Source: CAD feature listing. Evaluate the final solid. Frame: model axes, mm. A direction names the side the tool comes from. Coordinates: 2 decimals unless noted, no trailing zeros. Write each loop counter-clockwise with the first axis right and the second up, starting at its lowest first coordinate (ties: lowest second). Pieces come first, ordered by that corner, then holes. Notation, with made-up numbers: (-23, -0.5) - (22, -0.5) arc R38 cw to (22, 37.5) - close; hole circle Ø7 at (15, 81.5). An arc over 180 degrees is marked (long way). One line per question, with ' | ' between items.
from build123d import *

# Parameters (mm, degrees)
SCHIZZO1_R                   = 10
SCHIZZO1_R_2                 = 1.2
ESTRUSIONE_ESTRUSIONE1_DEPTH = 6
SCHIZZO2_R                   = 5
ESTRUSIONE_ESTRUSIONE2_DEPTH = 53
SCHIZZO9_W                   = 4
SCHIZZO9_H                   = 2.3
SMUSSO3_SIZE                 = 0.3
FORO_8_1_8_1_1_D             = 8.1
FORO_8_1_8_1_1_DEPTH         = 2
FORO_8_1_8_1_1_TIP           = 2.433485507
SMUSSO5_SIZE                 = 0.5
TAGLIO_ESTRUSIONE1_START     = -29
TAGLIO_ESTRUSIONE1_DEPTH     = 29
PREFORO_DA_MASCHIARE_M3_1_D  = 2.5
SMUSSO4_SIZE                 = 0.3
FORO_8_1_8_1_2_D             = 8.1
FORO_8_1_8_1_2_DEPTH         = 2.5
FORO_8_1_8_1_2_TIP           = 2.433485507
SCHIZZO17_W                  = 1.3
SCHIZZO17_H                  = 4.4
RACCORDO1_R                  = 0.2
SCHIZZO18_W                  = 0.2
SCHIZZO18_H                  = 1.1


with BuildPart() as part:
    # Schizzo1 → Estrusione-Estrusione1 (new body)
    with BuildSketch(Plane(origin=(0, 0, 0), x_dir=(1, 0, 0), z_dir=(0, 1, 0))):
        with Locations(Location((0, 0, 0), (0, 0, 270))):
            Circle(SCHIZZO1_R)
        with Locations(Location((0, 8, 0), (0, 0, 270))):
            Circle(SCHIZZO1_R_2, mode=Mode.SUBTRACT)
        with Locations(Location((5.656854249, 5.656854249, 0), (0, 0, 270))):
            Circle(SCHIZZO1_R_2, mode=Mode.SUBTRACT)
        with Locations(Location((8, 0, 0), (0, 0, 270))):
            Circle(SCHIZZO1_R_2, mode=Mode.SUBTRACT)
        with Locations(Location((5.656854249, -5.656854249, 0), (0, 0, 270))):
            Circle(SCHIZZO1_R_2, mode=Mode.SUBTRACT)
        with Locations(Location((0, -8, 0), (0, 0, 270))):
            Circle(SCHIZZO1_R_2, mode=Mode.SUBTRACT)
        with Locations(Location((-5.656854249, -5.656854249, 0), (0, 0, 270))):
            Circle(SCHIZZO1_R_2, mode=Mode.SUBTRACT)
        with Locations(Location((-8, 0, 0), (0, 0, 270))):
            Circle(SCHIZZO1_R_2, mode=Mode.SUBTRACT)
        with Locations(Location((-5.656854249, 5.656854249, 0), (0, 0, 270))):
            Circle(SCHIZZO1_R_2, mode=Mode.SUBTRACT)
    extrude(amount=ESTRUSIONE_ESTRUSIONE1_DEPTH)

    # Schizzo2 → Estrusione-Estrusione2 (add)
    with BuildSketch(Plane(origin=(0, 6, 0), x_dir=(1, 0, 0), z_dir=(0, 1, 0))):
        with Locations(Location((0, 0, 0), (0, 0, 270))):
            Circle(SCHIZZO2_R)
    extrude(amount=ESTRUSIONE_ESTRUSIONE2_DEPTH)

    # Schizzo9 → Taglia-Rivoluzione3 (revolve, cut)
    with BuildSketch(Plane.XY, mode=Mode.PRIVATE) as taglia_rivoluzione3_sk:
        with Locations((-8, 4.85)):
            Rectangle(SCHIZZO9_W, SCHIZZO9_H)
    revolve(taglia_rivoluzione3_sk.sketch.rotate(Axis((0, 0, 0), (0, 1, 0)), 270), axis=Axis((0, 0, 0), (0, 1, 0)), mode=Mode.SUBTRACT)

    # Smusso3
    smusso3_edges = [part.edges().sort_by_distance(p)[0] for p in [
        (0, 3.7, -10),
    ]]
    chamfer(smusso3_edges, length=SMUSSO3_SIZE)

    # Schizzo4 → Taglia-Rivoluzione2 (revolve, cut)
    with BuildSketch(Plane.XY, mode=Mode.PRIVATE) as taglia_rivoluzione2_sk:
        with BuildLine():
            Line((-5, 8), (-4.813629669, 7.304456457))
            ThreePointArc((-4.813629669, 7.304456457), (-4.803422055, 7.253139316), (-4.8, 7.200928839))
            Line((-4.8, 7.200928839), (-4.8, 6.4))
            ThreePointArc((-4.8, 6.4), (-4.917157288, 6.117157288), (-5.2, 6))
            Line((-5.2, 6), (-7, 6))
            Line((-7, 6), (-7, 8))
            Line((-7, 8), (-5, 8))
        make_face()
    revolve(taglia_rivoluzione2_sk.sketch.rotate(Axis((0, 0, 0), (0, 1, 0)), 270), axis=Axis((0, 0, 0), (0, 1, 0)), mode=Mode.SUBTRACT)

    # Foro Ø8.1 (8.1)-1
    with Locations(Plane.XZ):
        with Locations((0, 0)):
            Hole(FORO_8_1_8_1_1_D / 2, depth=FORO_8_1_8_1_1_DEPTH)
            with Locations((0, 0, -(FORO_8_1_8_1_1_DEPTH + FORO_8_1_8_1_1_TIP / 2))):  # 118° drill point
                Cone(0, FORO_8_1_8_1_1_D / 2, FORO_8_1_8_1_1_TIP, mode=Mode.SUBTRACT)

    # Smusso5
    smusso5_edges = [part.edges().sort_by_distance(p)[0] for p in [
        (0, 59, -5),
    ]]
    chamfer(smusso5_edges, length=SMUSSO5_SIZE)

    # Schizzo10 → Taglio-Estrusione1 (cut)
    with BuildSketch(Plane(origin=(0, 59, 0), x_dir=(1, 0, 0), z_dir=(0, 1, 0)).offset(TAGLIO_ESTRUSIONE1_START)):
        with BuildLine():
            Line((3.5, -3.570714214), (3.5, 3.570714214))
            ThreePointArc((3.5, 3.570714214), (5, 0), (3.5, -3.570714214))
        make_face()
    extrude(amount=TAGLIO_ESTRUSIONE1_DEPTH, mode=Mode.SUBTRACT)

    # Preforo da maschiare M3-1 (through all)
    with Locations(Plane(origin=(3.5, 0, 0), x_dir=(0, 0, -1), z_dir=(1, 0, 0))):
        with Locations((0, 44)):
            Hole(PREFORO_DA_MASCHIARE_M3_1_D / 2)

    # Smusso4
    smusso4_edges = [part.edges().sort_by_distance(p)[0] for p in [
        (3.5, 44, -1.25),
    ]]
    chamfer(smusso4_edges, length=SMUSSO4_SIZE)

    # Foro Ø8.1 (8.1)-2
    with Locations(Plane.XZ):
        with Locations((0, 0)):
            Hole(FORO_8_1_8_1_2_D / 2, depth=FORO_8_1_8_1_2_DEPTH)
            with Locations((0, 0, -(FORO_8_1_8_1_2_DEPTH + FORO_8_1_8_1_2_TIP / 2))):  # 118° drill point
                Cone(0, FORO_8_1_8_1_2_D / 2, FORO_8_1_8_1_2_TIP, mode=Mode.SUBTRACT)

    # Schizzo17 → Taglia-Rivoluzione4 (revolve, cut)
    with BuildSketch(Plane.XY, mode=Mode.PRIVATE) as taglia_rivoluzione4_sk:
        with Locations((-4.35, 15.4)):
            Rectangle(SCHIZZO17_W, SCHIZZO17_H)
    revolve(taglia_rivoluzione4_sk.sketch.rotate(Axis((0, 0, 0), (0, 1, 0)), 270), axis=Axis((0, 0, 0), (0, 1, 0)), mode=Mode.SUBTRACT)

    # Raccordo1
    raccordo1_edges = [part.edges().sort_by_distance(p)[0] for p in [
        (0, 13.2, 3.7),
        (0, 17.6, 3.7),
    ]]
    fillet(raccordo1_edges, radius=RACCORDO1_R)

    # Schizzo18 → Taglia-Rivoluzione5 (revolve, cut)
    with BuildSketch(Plane.XY, mode=Mode.PRIVATE) as taglia_rivoluzione5_sk:
        with Locations((-4.9, 25.45)):
            Rectangle(SCHIZZO18_W, SCHIZZO18_H)
    revolve(taglia_rivoluzione5_sk.sketch.rotate(Axis((0, 0, 0), (0, 1, 0)), 270), axis=Axis((0, 0, 0), (0, 1, 0)), mode=Mode.SUBTRACT)


solid = part.part
Item 1: Access query for faces 1 (the face through (-9.76, 1.68, -2.17)), 2 (the face through (-4.88, 42.02, -1.08)), 3 (the face through (0.1, 0, 4.3)), 4 (the face through (0.878, 1.268, -3.954)), 5 (the face through (3.612, 15.428, 0.802)). Directions: +Z, -Z, +X, -X, +Y, -Y. A direction counts if a zero-diameter tool reaches every point of the face in a straight line with its end or side. Return the directions, or none.
Check sheet entries:
face 1: +Y, -Y | face 2: +Y | face 3: +Z, -Z, +X, -X, -Y | face 4: -Y | face 5: none
Item 2: Cut plane C-C on y = 55.5. Return loops of the section in (x, z), and give its area (3 significant figures).
Check sheet entries:
outline: (3.5, -3.57) - (3.5, 3.57) arc R5 ccw (long way) to start | area: 71.2 mm²
Item 3: Ray query, line 1 along Z through (x, y) = (0, 0.6); line 2 along Z through (x, y) = (-2.25, 44). Return the intervals inside material, ascending. Write a range as [from, to].
Check sheet entries:
line 1: [-10, -9.2], [-6.8, -4.05], [4.05, 6.8], [9.2, 10] | line 2: [-4.47, -1.25], [1.25, 4.47]
Item 4: Cut plane B-B on y = 15. Return loops of the section in (x, z).
Check sheet entries:
outline: circle Ø7.4 at (0, 0)
Item 5: Pin query (flat end, axial travel): pin 1 Ø2 at (y, z) = (17, 4.5) entering from +X; pin 2 Ø2 at (x, y) = (4.5, 24.5) entering from -Z; pin 3 Ø10 at (y, z) = (39, -6.5) entering from -X; pin 4 Ø1.5 at (x, y) = (5.5, 40.5) entering from +Z. Return the tip coordinate at first contact, or that it passes through.
Check sheet entries:
pin 1: x = 3.36 | pin 2: z = -3.57 | pin 3: x = -4.77 | pin 4: through
Item 6: Mould query, pull axis X, two halves, no side actions, for faces 6 (the face through (-1.802, 4.866, -5.723)), 7 (the face through (0.05, 1.82, 6.8)), 8 (the face through (3, 13.2, -3)). Classes: pulls with the +X half, pulls with the -X half, needs draft (parallel to the pull), parting line crosses it, or undercut.
Check sheet entries:
face 6: parting line crosses it | face 7: undercut | face 8: needs draft
Item 7: Cut plane A-A on y = 44. Return loops of the section in (x, z), and give its area (3 significant figures).
Check sheet entries:
outline: (-4.84, -1.25) arc R5 ccw to (3.5, -3.57) - (3.5, -1.55) - (3.2, -1.25) - close; (-4.84, 1.25) - (3.2, 1.25) - (3.5, 1.55) - (3.5, 3.57) arc R5 ccw to start | area: 49.9 mm²
